```python
from build123d import *

# Parameters (mm, degrees)
BASESBEAM_DEPTH = 457.2
TOEFILLET_R     = 2.794


with BuildPart() as part:
    # Sketch1 → BaseSbeam (new body, symmetric)
    with BuildSketch(Plane.XY):
        with BuildLine():
            Line((0, 0), (0, 4.82792597))
            Line((0, 4.82792597), (25.214048892, 9.030574012))
            ThreePointArc((25.214048892, 9.030574012), (29.623433353, 11.535173088), (31.369, 16.296337329))
            Line((31.369, 16.296337329), (31.369, 85.303662671))
            ThreePointArc((31.369, 85.303662671), (29.623433353, 90.064826912), (25.214048892, 92.569425988))
            Line((25.214048892, 92.569425988), (0, 96.77207403))
            Line((0, 96.77207403), (0, 101.6))
            Line((0, 101.6), (67.6402, 101.6))
            Line((67.6402, 101.6), (67.6402, 96.77207403))
            Line((67.6402, 96.77207403), (42.426151108, 92.569425988))
            ThreePointArc((42.426151108, 92.569425988), (38.016766647, 90.064826912), (36.2712, 85.303662671))
            Line((36.2712, 85.303662671), (36.2712, 16.296337329))
            ThreePointArc((36.2712, 16.296337329), (38.016766647, 11.535173088), (42.426151108, 9.030574012))
            Line((42.426151108, 9.030574012), (67.6402, 4.82792597))
            Line((67.6402, 4.82792597), (67.6402, 0))
            Line((67.6402, 0), (0, 0))
        make_face()
    extrude(amount=BASESBEAM_DEPTH, both=True)

    # ToeFillet
    toefillet_edges = [part.edges().sort_by_distance(p)[0] for p in [
        (67.6402, 4.82792597, 0),
        (67.6402, 96.77207403, 0),
        (0, 96.77207403, 0),
        (0, 4.82792597, 0),
    ]]
    fillet(toefillet_edges, radius=TOEFILLET_R)


solid = part.part
```
Here's how the part is built. I have some questions about the finished solid (model axes, mm). A direction names the side the tool comes from. Coordinates: 2 decimals unless noted, no trailing zeros. Loops run counter-clockwise (first coordinate to the right, second up) from the corner with the lowest first, then second, coordinate; pieces in that order, holes last. Notation, with made-up numbers: M 6.25,25 L 16.25,25 A23 cw 16.25,56 Z; hole C 52.5,-4 d6. An arc over 180 degrees is marked long. One line per item, written item: value.
1. Will these pins go through, and if not, where does the flat tip stop? pin 1 Ø1.5 at (y, z) = (16, -207) entering from -X; pin 2 Ø20.5 at (y, z) = (44, 106.5) entering from +X; pin 3 Ø10 at (y, z) = (38, 3) entering from -X.
Geometry says:
pin 1: stops at x = 31.29
pin 2: stops at x = 36.27
pin 3: stops at x = 31.37
2. Imagine slicing it at A-A (x = 10.5). List the corners of the cut face in (y, z) for me.
Geometry says:
outline: M 0,-457.2 L 6.58,-457.2 L 6.58,457.2 L 0,457.2 Z; M 95.02,-457.2 L 101.6,-457.2 L 101.6,457.2 L 95.02,457.2 Z
3. Imagine slicing it at C-C (y = 38). List the corners of the cut face in (x, z) for me.
Geometry says:
outline: M 31.37,-457.2 L 36.27,-457.2 L 36.27,457.2 L 31.37,457.2 Z
4. Imagine slicing it at B-B (z = 317). List the corners of the cut face in (x, y) for me, and give its area (3 significant figures).
Geometry says:
outline: M 0,0 L 67.64,0 L 67.64,2.46 A2.79 ccw 65.31,5.22 L 42.43,9.03 A7.37 cw 36.27,16.3 L 36.27,85.3 A7.37 cw 42.43,92.57 L 65.31,96.38 A2.79 ccw 67.64,99.14 L 67.64,101.6 L 0,101.6 L 0,99.14 A2.79 ccw 2.33,96.38 L 25.21,92.57 A7.37 cw 31.37,85.3 L 31.37,16.3 A7.37 cw 25.21,9.03 L 2.33,5.22 A2.79 ccw 0,2.46 Z
area: 1,460 mm2
5. Thinking about a two-plate mould opening in Y: for faces 1 (the flat face through (33, 101.6, 6)), 2 (the flat face through (53.71, 7.15, 6.4)), 3 (the flat face through (34, 51, 457.2)), which applies, +Y half, -Y half, draft (parallel to the pull), parting line (faces both ways), or undercut?
Geometry says:
face 1: +Y half
face 2: undercut
face 3: draft
6. Please list where these lines run through material, in increasing order: probe 1 along Y at (x, z) = (42, 374); probe 2 along X at (y, z) = (69, -142.5); probe 3 along Y at (x, z) = (18, 190.5).
Geometry says:
probe 1: y = 0 to 9.11, 92.49 to 101.6
probe 2: x = 31.37 to 36.27
probe 3: y = 0 to 7.83, 93.77 to 101.6
7. On a 3-axis mill with a long thin cutter (end or side, diameter ignored), from which of +Z, -Z, +X, -X, +Y, -Y can I reach the whole of each face in a straight line? I mean faces 4 (the flat face through (13.93, 94.45, 6.4)), 5 (the flat face through (36.271, 51, 6)), 6 (the flat face through (34, 0, 6)). Say none if no direction works.
Geometry says:
face 4: +Z, -Z, -X
face 5: +Z, -Z, +X
face 6: +Z, -Z, +X, -X, -Y
